Geometry: final body of the model. Coordinates: model frame, mm. Face numbers are marked on the shaded views. Give positions to 0.01 mm unless a question says otherwise; leave off trailing zeros. Write each loop counter-clockwise with the first axis right and the second up, starting at its lowest first coordinate (ties: lowest second). Pieces come first, ordered by that corner, then holes.
Q1. Cut plane B-B on y = 22.25. Count the separate pieces of the cut face and the enclosed holes in it, plus the area to 3 significant figures.
Q2. Cut plane A-A on z = 13.5. Return the cut outline in (x, y), plus the area to 3 significant figures.
Q3. Cut plane D-D on x = -29. Return the cut outline in (y, z).
Q4. Cut plane C-C on z = 56.5. Return the cut outline in (x, y).
Q5. Line query: L1, parallel to Z at x = -24, y = 17; L2, parallel to X at y = 27, z = 31.5; L3, parallel to Z at x = -42, y = 15. Output: solid intervals per line, ascending.
Q6. Pin query (flat end, axial travel): pin 1 (2 mm diameter, centred on x = -23, y = 26.5, fed in from -Z); pin 2 (4 mm diameter, centred on x = -27.5, z = 3, fed in from +Y); pin 3 (1 mm diameter, centred on x = -41, z = 12.5, fed in from +Y); pin 4 (5 mm diameter, centred on x = -34, y = 18, fed in from +Z). Return the tip coordinate at first contact, or that it passes through.
Q7. Draft query along X for the marked faces 1, 2 and 3. Return one class per face: pulls with the +X half, pulls with the -X half, needs draft (parallel to the pull), parting line crosses it, or undercut.
```python
from build123d import *

# Parameters (mm, degrees)
F0_R      = 3.5
F1_DEPTH  = 5
F2_R      = 9.99999
F4_START  = 5
F3_W      = 5
F3_H      = 20
F4_DEPTH  = 76
F5_R      = 3.5
F6_DEPTH  = 79.3
F7_R      = 9.99999
F8_DEPTH  = 16.5
F3_W_2    = 7
F9_DEPTH  = 10
F10_SIZE  = 6.99999
F11_DEPTH = 55.6


# Not quite as in the source:
# - a fillet or chamfer is up to 0.001 mm smaller than in the source, because OpenCascade refuses the exact size


with BuildPart() as f1:
    # F0 (on Top) → F1 (new body)
    with BuildSketch(Plane.XY):
        with BuildLine():
            Line((-36.1016022205, 30.0462352857), (-46.2016022205, 30.0462352857))
            Line((-46.2016022205, 30.0462352857), (-46.2016022205, 10.0462352857))
            Line((-46.2016022205, 10.0462352857), (-36.1016022205, 10.0462352857))
            ThreePointArc((-36.1016022205, 10.0462352857), (-46.1016022205, 20.0462352857), (-36.1016022205, 30.0462352857))
        make_face()
        with BuildLine():
            Line((-11.2016022205, 30.0462352857), (-36.1016022205, 30.0462352857))
            ThreePointArc((-36.1016022205, 30.0462352857), (-29.0305344087, 27.1173030976), (-26.1016022205, 20.0462352857))
            ThreePointArc((-26.1016022205, 20.0462352857), (-29.0305344087, 12.9751674738), (-36.1016022205, 10.0462352857))
            Line((-36.1016022205, 10.0462352857), (-11.2016022205, 10.0462352857))
            Line((-11.2016022205, 10.0462352857), (-11.2016022205, 30.0462352857))
        make_face()
        with BuildLine():
            ThreePointArc((-26.1016022205, 20.0462352857), (-29.0305344087, 27.1173030976), (-36.1016022205, 30.0462352857))
            ThreePointArc((-36.1016022205, 30.0462352857), (-46.1016022205, 20.0462352857), (-36.1016022205, 10.0462352857))
            ThreePointArc((-36.1016022205, 10.0462352857), (-29.0305344087, 12.9751674738), (-26.1016022205, 20.0462352857))
        make_face()
        with Locations((-36.1016022205, 20.0462352857)):
            Circle(F0_R, mode=Mode.SUBTRACT)
    extrude(amount=F1_DEPTH)

    # F2 (radius 10 in the source; OpenCascade refuses exactly that, so slightly less here)
    f2_edges = [f1.edges().sort_by_distance(p)[0] for p in [
        (-46.201602, 30.046235, 2.5),
        (-46.201602, 10.046235, 2.5),
    ]]
    fillet(f2_edges, radius=F2_R)

    # F3 (on Top) → F4 (join)
    with BuildSketch(Plane.XY.offset(F4_START)):
        with Locations((-13.7016022205, 20.0760087371)):
            Rectangle(F3_W, F3_H)
    extrude(amount=F4_DEPTH)

    # F5 (on Right) → F6 (cut)
    with BuildSketch(Plane.YZ):
        with Locations((20.2629771084, 71.5329723358)):
            Circle(F5_R)
    extrude(amount=F6_DEPTH, mode=Mode.SUBTRACT)

    # F7 (radius 10 in the source; OpenCascade refuses exactly that, so slightly less here)
    f7_edges = [f1.edges().sort_by_distance(p)[0] for p in [
        (-13.701602, 10.076009, 81),
        (-13.701602, 30.076009, 81),
    ]]
    fillet(f7_edges, radius=F7_R)

    # F0 (on Top) → F8 (join)
    with BuildSketch(Plane.XY):
        with BuildLine():
            ThreePointArc((-26.1016022205, 20.0462352857), (-29.0305344087, 27.1173030976), (-36.1016022205, 30.0462352857))
            ThreePointArc((-36.1016022205, 30.0462352857), (-46.1016022205, 20.0462352857), (-36.1016022205, 10.0462352857))
            ThreePointArc((-36.1016022205, 10.0462352857), (-29.0305344087, 12.9751674738), (-26.1016022205, 20.0462352857))
        make_face()
        with Locations((-36.1016022205, 20.0462352857)):
            Circle(F0_R, mode=Mode.SUBTRACT)
    extrude(amount=F8_DEPTH)

    # F3 (on Top) → F9 (join)
    with BuildSketch(Plane.XY):
        with Locations((-13.7016022205, 20.0760087371)):
            Rectangle(F3_W, F3_H)
        with Locations((-19.7016022205, 20.0760087371)):
            Rectangle(F3_W_2, F3_H)
    extrude(amount=F9_DEPTH)

    # F10 (size 7 in the source; OpenCascade refuses exactly that, so slightly less here)
    f10_edges = [f1.edges().sort_by_distance(p)[0] for p in [
        (-23.201602, 20.076009, 10),
    ]]
    chamfer(f10_edges, length=F10_SIZE)

    # F5 (on Right) → F11 (cut)
    with BuildSketch(Plane.YZ):
        with Locations((20.2629771084, 71.5329723358)):
            Circle(F5_R)
    extrude(amount=-F11_DEPTH, mode=Mode.SUBTRACT)


solid = f1.part
```
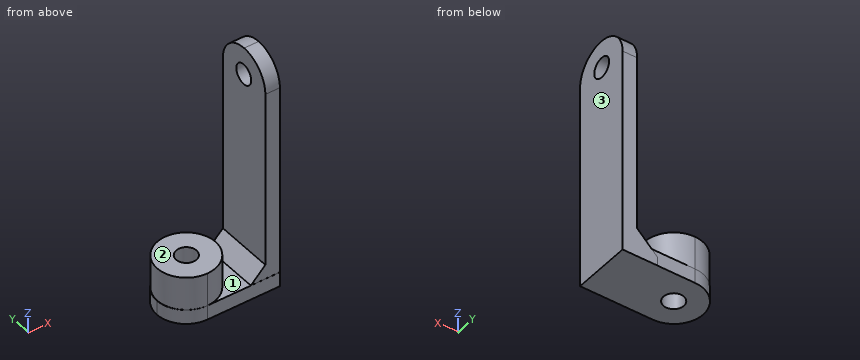
Data:
1. separate pieces: 3
1. enclosed holes: 0
1. area: 671 mm2
2. outline: circle Ø20 at (-36.1, 20.05); (-16.2, 10.08) - (-11.2, 10.08) - (-11.2, 30.08) - (-16.2, 30.08) - close; hole circle Ø7 at (-36.1, 20.05)
2. area: 376 mm2
3. outline: (10.05, 0) - (30.05, 0) - (30.05, 5) - (27.09, 5) - (27.09, 16.5) - (13.01, 16.5) - (13.01, 5) - (10.05, 5) - close
4. outline: (-16.2, 10.08) - (-11.2, 10.08) - (-11.2, 30.08) - (-16.2, 30.08) - close
5. L1: z = 0 to 5
5. L2: x = -16.2 to -11.2
5. L3: z = 0 to 16.5
6. pin 1: stops at z = 0
6. pin 2: stops at y = 30.05
6. pin 3: stops at y = 29.03
6. pin 4: stops at z = 16.5
7. face 1: undercut
7. face 2: needs draft
7. face 3: pulls with the +X half
